from build123d import *

# Parameters (mm, degrees)
F0_R            = 20
F1_DEPTH        = 10
F3_DEPTH        = 8.5
F4_R            = 2
F5_DEPTH        = 10.001
F5_COPIES_COUNT = 6
F7_DEPTH        = 3.25
F7_COPIES_COUNT = 6
F8_R            = 5.08
F9_DEPTH        = 10.001


# Not quite as in the source:
# - a pattern or mirror of a feature is missing from the dataset's text; its kind, count and spacing are read off the source's solid


with BuildPart() as f1:
    # F0 (on Front) → F1 (new body)
    with BuildSketch(Plane.XZ):
        Circle(F0_R)
    extrude(amount=F1_DEPTH)

    # F2 (on face) → F3 (cut)
    with BuildSketch(Plane(origin=(0, 0, 0), x_dir=(-1, 0, 0), z_dir=(0, 1, 0))):
        Polygon((3.3197640478, 5.75), (-3.3197640478, 5.75), (-6.6395280957, 0), (-3.3197640478, -5.75), (3.3197640478, -5.75), (6.6395280957, 0), align=None)
    extrude(amount=-F3_DEPTH, mode=Mode.SUBTRACT)

    # F4 (on face) → F5 (cut, through all)
    with BuildSketch(Plane.XZ.offset(10)):
        with Locations((0, 15)):
            Circle(F4_R)
    f5 = extrude(amount=-F5_DEPTH, mode=Mode.SUBTRACT)

    # F5_copies: F5 ×6 about axis
    f5_copies_axis = Axis((0, 0, 0), (0, 1, 0))
    for i in range(1, F5_COPIES_COUNT):
        add(f5.rotate(f5_copies_axis, i * 360 / F5_COPIES_COUNT), mode=Mode.SUBTRACT)

    # F6 (on face) → F7 (cut)
    with BuildSketch(Plane.XZ.offset(10)):
        Polygon((2.375, 19.113620668), (-2.375, 19.113620668), (-4.75, 15), (-2.375, 10.886379332), (2.375, 10.886379332), (4.75, 15), align=None)
    f7 = extrude(amount=-F7_DEPTH, mode=Mode.SUBTRACT)

    # F7_copies: F7 ×6 about axis
    f7_copies_axis = Axis((0, 0, 0), (0, 1, 0))
    for i in range(1, F7_COPIES_COUNT):
        add(f7.rotate(f7_copies_axis, i * 360 / F7_COPIES_COUNT), mode=Mode.SUBTRACT)

    # F8 (on face) → F9 (cut, through all)
    with BuildSketch(Plane.XZ.offset(10)):
        Circle(F8_R)
    extrude(amount=-F9_DEPTH, mode=Mode.SUBTRACT)


solid = f1.part
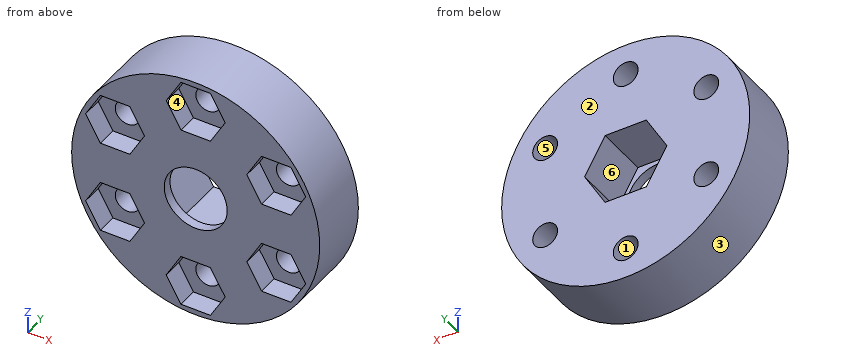
Can you work these out from the model? Positions are in its coordinate system, mm. Face numbers are marked on the shaded views. A direction names the side the tool comes from. Round coordinates to 2 decimals unless told otherwise and drop trailing zeros. Write each loop counter-clockwise with the first axis right and the second up, starting at its lowest first coordinate (ties: lowest second). Pieces come first, ordered by that corner, then holes. Notation, with made-up numbers: (-15, 81) - (13, 81) arc R11 cw to (13, 98) - close; hole circle Ø1 at (58, 76.5). An arc over 180 degrees is marked (long way). Write each question's results on one line, items separated by ' | '. Start each with the question number.
1) Suppose I cut it at D-D (x = -13.5). List the corners of the cut face in (y, z) for me, and give its area (3 significant figures).
2) For pin 1 Ø2.5 at (x, y) = (14, -9) entering from +Z; pin 2 Ø4 at (x, y) = (8, -6) entering from +Z; pin 3 Ø3.5 at (x, y) = (13, -7.5) entering from -Z; pin 4 Ø3 at (x, z) = (12.99, -7.5) entering from +Y, each with a flat end and sliding along its axis, tell me the tip position at first contact or that it passes through.
3) Suppose I cut it at B-B (z = -2). List the corners of the cut face in (x, y) for me, and give its area (3 significant figures).
4) Please list where these lines run through material, in increasing order: line 1 (Z direction, x = 0, y = -9.35); line 2 (Z direction, x = 0, y = -5.25); line 3 (X direction, y = -3, z = 9).
5) We'd pull the mould along X, two halves only. Please class the marked faces 1, 2 and 3: released by +X, released by -X, zero draft, split by the parting line, or undercut.
6) Suppose I cut it at A-A (x = 0). List the corners of the cut face in (y, z) for me, and give its area (3 significant figures).
7) Which directions (+Z, -Z, +X, -X, +Y, -Y) give clear straight access to the entire face, cutting with the end or side of a thin tool? Please do the marked faces 4, 5 and 6.
8) Suppose I cut it at C-C (y = -5.75). List the corners of the cut face in (x, z) for me, and give its area (3 significant figures).
Here are the results:
1) outline: (-10, -14.76) - (0, -14.76) - (0, -9.43) - (-6.75, -9.43) - (-6.75, -11.61) - (-10, -11.61) - close; (-10, -3.39) - (-6.75, -3.39) - (-6.75, -5.57) - (0, -5.57) - (0, 5.57) - (-6.75, 5.57) - (-6.75, 3.39) - (-10, 3.39) - close; (-10, 11.61) - (-6.75, 11.61) - (-6.75, 9.43) - (0, 9.43) - (0, 14.76) - (-10, 14.76) - close | area: 189 mm2
2) pin 1: stops at z = 15.41 | pin 2: stops at z = 19.08 | pin 3: stops at z = -16.54 | pin 4: passes through
3) outline: (-19.9, -10) - (-4.67, -10) - (-4.67, -8.5) - (-5.48, -8.5) - (-5.48, 0) - (-19.9, 0) - close; (4.67, -10) - (19.9, -10) - (19.9, 0) - (5.48, 0) - (5.48, -8.5) - (4.67, -8.5) - close | area: 291 mm2
4) line 1: z = -20 to -19.11, -10.89 to -5.08, 5.08 to 10.89, 19.11 to 20 | line 2: z = -20 to -17, -13 to -5.75, 5.75 to 13, 17 to 20 | line 3: x = -17.86 to -14.31, -11.67 to 11.67, 14.31 to 17.86
5) face 1: undercut | face 2: zero draft | face 3: split by the parting line
6) outline: (-10, -20) - (0, -20) - (0, -17) - (-6.75, -17) - (-6.75, -19.11) - (-10, -19.11) - close; (-10, -10.89) - (-6.75, -10.89) - (-6.75, -13) - (0, -13) - (0, -5.75) - (-8.5, -5.75) - (-8.5, -5.08) - (-10, -5.08) - close; (-10, 5.08) - (-8.5, 5.08) - (-8.5, 5.75) - (0, 5.75) - (0, 13) - (-6.75, 13) - (-6.75, 10.89) - (-10, 10.89) - close; (-10, 19.11) - (-6.75, 19.11) - (-6.75, 17) - (0, 17) - (0, 20) - (-10, 20) - close | area: 180 mm2
7) face 4: -Y | face 5: +Y, -Y | face 6: +Y
8) outline: circle Ø40 at (0, 0); hole circle Ø4 at (-12.99, -7.5); hole circle Ø4 at (-12.99, 7.5); hole (-6.64, 0) - (-3.32, -5.75) - (3.32, -5.75) - (6.64, 0) - (3.32, 5.75) - (-3.32, 5.75) - close; hole circle Ø4 at (0, -15); hole circle Ø4 at (0, 15); hole circle Ø4 at (12.99, -7.5); hole circle Ø4 at (12.99, 7.5) | area: 1,070 mm2
